from build123d import *

# Parameters (mm, degrees)
SKETCH1_R           = 29
BOSS_EXTRUDE1_DEPTH = 90
SKETCH2_R           = 25.5
BOSS_EXTRUDE3_DEPTH = 65
BOSS_EXTRUDE3_TAPER = 10
SKETCH4_R           = 5
BOSS_EXTRUDE4_DEPTH = 13
SKETCH10_R          = 30
BOSS_EXTRUDE5_DEPTH = 70
BOSS_EXTRUDE5_TAPER = -8
SKETCH11_R          = 40.837858429
BOSS_EXTRUDE6_DEPTH = 10
SKETCH12_R          = 5
BOSS_EXTRUDE7_DEPTH = 20
BOSS_EXTRUDE7_TAPER = 4
SKETCH14_R          = 2
BOSS_EXTRUDE8_DEPTH = 30


with BuildPart() as part:
    # Sketch1 → Boss-Extrude1 (new body)
    with BuildSketch(Plane(origin=(0, 0, 0), x_dir=(1, 0, 0), z_dir=(0, 1, 0))):
        Circle(SKETCH1_R)
    extrude(amount=BOSS_EXTRUDE1_DEPTH)

    # Sketch2 → Boss-Extrude3 (add)
    with BuildSketch(Plane(origin=(0, 90, 0), x_dir=(1, 0, 0), z_dir=(0, 1, 0))):
        Circle(SKETCH2_R)
    extrude(amount=BOSS_EXTRUDE3_DEPTH, taper=BOSS_EXTRUDE3_TAPER)

    # Sketch4 → Boss-Extrude4 (add)
    with BuildSketch(Plane(origin=(0, 155, 0), x_dir=(1, 0, 0), z_dir=(0, 1, 0))):
        Circle(SKETCH4_R)
    extrude(amount=BOSS_EXTRUDE4_DEPTH)

    # Sketch10 → Boss-Extrude5 (add)
    with BuildSketch(Plane.XZ):
        Circle(SKETCH10_R)
    extrude(amount=BOSS_EXTRUDE5_DEPTH, taper=BOSS_EXTRUDE5_TAPER)

    # Sketch11 → Boss-Extrude6 (add)
    with BuildSketch(Plane.XZ.offset(70)):
        Circle(SKETCH11_R)
    extrude(amount=BOSS_EXTRUDE6_DEPTH)

    # Sketch12 → Boss-Extrude7 (add)
    with BuildSketch(Plane.XZ.offset(80)):
        with Locations((26.346299314, 13.003540379)):
            Circle(SKETCH12_R)
    extrude(amount=BOSS_EXTRUDE7_DEPTH, taper=BOSS_EXTRUDE7_TAPER)

    # Sketch14 → Boss-Extrude8 (add)
    with BuildSketch(Plane.XZ.offset(100)):
        with Locations((26.346299314, 13.003540379)):
            Circle(SKETCH14_R)
    extrude(amount=BOSS_EXTRUDE8_DEPTH)


solid = part.part
Read the model definition and answer for the solid it produces. Units are mm, in the model's axes. A direction names the side the tool comes from. Round coordinates to 2 decimals unless told otherwise and drop trailing zeros. Write each loop counter-clockwise with the first axis right and the second up, starting at its lowest first coordinate (ties: lowest second). Pieces come first, ordered by that corner, then holes. Notation, with made-up numbers: (-17.75, 56) - (14.25, 56) arc R12 cw to (14.25, 69) - close; hole circle Ø5 at (79, 52.25). An arc over 180 degrees is marked (long way). Use a Markdown table: item, result.
(1) The part is cut by section A-A (x = 0). Write down the section's boundary in (y, z), then the cut area to 3 significant figures.
Reported:
| item | result |
|---|---|
| outline | (-80, -40.84) - (-70, -40.84) - (-70, -39.84) - (0, -30) - (0, -29) - (90, -29) - (90, -25.5) - (155, -14.04) - (155, -5) - (168, -5) - (168, 5) - (155, 5) - (155, 14.04) - (90, 25.5) - (90, 29) - (0, 29) - (0, 30) - (-70, 39.84) - (-70, 40.84) - (-80, 40.84) - close |
| area | 13,600 mm2 |
(2) Each of these flat-tipped pins is pushed along its axis until it touches: pin 1 Ø10 at (y, z) = (-74, -19.5) entering from -X; pin 2 Ø10 at (x, z) = (-8, -21) entering from -Y; pin 3 Ø3 at (y, z) = (76, -20) entering from -X. Where does it stop, or does it pass through?
Reported:
| item | result |
|---|---|
| pin 1 | x = -38.18 |
| pin 2 | y = -80 |
| pin 3 | x = -22.33 |
(3) Which of the six approach directions +Z, -Z, +X, -X, +Y, -Y give full straight-line access (tool end or side, diameter ignored) to faces 1 (the flat face through (28, -100, 11)), 2 (the cylindrical face through (-8.853, -74.93, -39.867)), 3 (the flat face through (0, 90, 26))?
Reported:
| item | result |
|---|---|
| face 1 | -Y |
| face 2 | +Y, -Y |
| face 3 | +Y |
(4) Straight lines are drawn through the part: line 1 along Z through (x, y) = (0.5, 43.5); line 2 along Z through (x, y) = (-26, -63.5); line 3 along Y through (x, z) = (1, 10). For each, find the intervals that lie inside material, in ascending order. Write a range as [from, to].
Reported:
| item | result |
|---|---|
| line 1 | [-29, 29] |
| line 2 | [-28.97, 28.97] |
| line 3 | [-80, 155] |
(5) The part is cut by section B-B (y = -29). Write down the section's boundary in (x, z), then the cut area to 3 significant figures.
Reported:
| item | result |
|---|---|
| outline | circle Ø68.15 at (0, 0) |
| area | 3,650 mm2 |
